from build123d import *

# Parameters (mm, degrees)
ESQUISSE1_R                  = 5
ESQUISSE1_R_2                = 4
ESQUISSE1_R_3                = 2
BOSS_EXTRU_1_DEPTH           = 5
ENL_V_MAT_EXTRU_1_DEPTH      = 1
ENL_V_MAT_EXTRU_1_DEPTH_BACK = 5
CONG_1_R                     = 10
ESQUISSE3_W                  = 20
ESQUISSE3_H                  = 5
BOSS_EXTRU_2_DEPTH           = 5
D_GAGEMENT_M21_D             = 2.4
D_GAGEMENT_M21_DEPTH         = 5
CONG_2_R                     = 10


with BuildPart() as part:
    # Esquisse1 → Boss.-Extru.1 (new body)
    with BuildSketch(Plane.XY):
        Polygon((0, 0), (30, 50), (50, 50), (50, 40), align=None)
        with Locations((36.602361653, 43.673429465)):
            Circle(ESQUISSE1_R, mode=Mode.SUBTRACT)
        with Locations((26.397486101, 32.05434035)):
            Circle(ESQUISSE1_R_2, mode=Mode.SUBTRACT)
        with Locations((18.668376917, 21.496804042)):
            Circle(ESQUISSE1_R_3, mode=Mode.SUBTRACT)
    extrude(amount=BOSS_EXTRU_1_DEPTH)

    # Esquisse2 → Enlèv. mat.-Extru.1 (cut, two sides)
    with BuildSketch(Plane(origin=(0, 0, 0), x_dir=(-1, 0, 0), z_dir=(0, 0, -1))) as enl_v_mat_extru_1_sk:
        with BuildLine():
            Line((0, 0), (-2.185666909, 3.642778182))
            ThreePointArc((-2.185666909, 3.642778182), (-2.607581993, 2.90339912), (-3.446178626, 2.756942901))
            Line((-3.446178626, 2.756942901), (0, 0))
        make_face()
    extrude(amount=ENL_V_MAT_EXTRU_1_DEPTH, mode=Mode.SUBTRACT)
    extrude(enl_v_mat_extru_1_sk.sketch, amount=-ENL_V_MAT_EXTRU_1_DEPTH_BACK, mode=Mode.SUBTRACT)

    # Congé1
    cong_1_edges = [part.edges().sort_by_distance(p)[0] for p in [
        (50, 40, 2.5),
    ]]
    fillet(cong_1_edges, radius=CONG_1_R)

    # Esquisse3 → Boss.-Extru.2 (add)
    with BuildSketch(Plane(origin=(0, 50, 0), x_dir=(1, 0, 0), z_dir=(0, 1, 0))):
        with Locations((40, -2.5)):
            Rectangle(ESQUISSE3_W, ESQUISSE3_H)
    extrude(amount=BOSS_EXTRU_2_DEPTH)

    # Dégagement M21
    with Locations(Plane.XY.offset(5)):
        with Locations((46, 52), (34, 52)):
            Hole(D_GAGEMENT_M21_D / 2, depth=D_GAGEMENT_M21_DEPTH)

    # Congé2
    cong_2_edges = [part.edges().sort_by_distance(p)[0] for p in [
        (30, 50, 2.5),
    ]]
    fillet(cong_2_edges, radius=CONG_2_R)


solid = part.part
Part model, mm, in its own coordinate system. A direction names the side the tool comes from. Round coordinates to 2 decimals unless told otherwise and drop trailing zeros. Write each loop counter-clockwise with the first axis right and the second up, starting at its lowest first coordinate (ties: lowest second). Pieces come first, ordered by that corner, then holes. Notation, with made-up numbers: M 7,78 L 24,78 A19 ccw 24,82 Z; hole C 88,-33.75 d4. An arc over 180 degrees is marked long. Return JSON: item names as keys, results as strings. Group by question number.
(1) Pin check, flat tips, straight feed: pin 1 Ø1.9 at (x, y) = (46, 52) entering from +Z; pin 2 Ø6.5 at (x, y) = (18.67, 21.5) entering from +Z; pin 3 Ø0.7 at (y, z) = (53.5, 1.5) entering from -X; pin 4 Ø2 at (x, z) = (7.5, 2.5) entering from -Y. Stop position of each tip, or through.
(2) Drill centre lines: probe 1 along Y at (x, z) = (33, 4.7); probe 2 along Y at (x, z) = (34, 1.8); probe 3 along Y at (x, z) = (32, 0.9). Where is each one in solid material? Low to high.
(3) Saw through at B-B on x = 28. Write the cut outline in (y, z).
(4) Saw through at A-A on y = 42. Write the cut outline in (x, z).
(5) Saw through at D-D on x = 33.5. Write the cut outline in (y, z), then the cut area to 3 significant figures.
(6) Saw through at C-C on z = 3.95. Write the cut outline in (x, y), then the cut area to 3 significant figures.
(7) Two-plate mould, pull along Y, no slides. Class faces 3 (the face through (31, 35, 5)), 4 (the face through (44.855, 52.36, 2.465)), 5 (the face through (25, 20, 2)): +Y half, -Y half, draft (parallel to the pull), parting line (faces both ways), or undercut.
(8) Which spindle directions (+Z, -Z, +X, -X, +Y, -Y) get a long thin tool onto all of the face, cutting with end or side? Do faces 1 (the face through (30, 54, 3)), 2 (the face through (31, 35, 0)). Say none if no direction does.
Returned:
{
 "1": {"pin 1": "through", "pin 2": "z = 5", "pin 3": "x = 30", "pin 4": "y = 5.2"},
 "2": {"probe 1": "26.4 to 40.21, 47.14 to 51.34, 52.66 to 55", "probe 2": "27.2 to 39.4, 47.94 to 50.8, 53.2 to 55", "probe 3": "25.6 to 41.72, 45.63 to 55"},
 "3": {"outline": "M 22.4,0 L 28.39,0 L 28.39,5 L 22.4,5 Z; M 35.72,0 L 46.67,0 L 46.67,5 L 35.72,5 Z"},
 "4": {"outline": "M 25.2,0 L 31.89,0 L 31.89,5 L 25.2,5 Z; M 41.31,0 L 49.6,0 L 49.6,5 L 41.31,5 Z"},
 "5": {"outline": "M 26.8,0 L 39.75,0 L 39.75,5 L 26.8,5 Z; M 47.59,0 L 50.91,0 L 50.91,5 L 47.59,5 Z; M 53.09,0 L 55,0 L 55,5 L 53.09,5 Z", "area": "90.9 mm²"},
 "6": {"outline": "M 2.19,3.64 A1 ccw 3.45,2.76 L 46.25,37 A10 ccw 50,44.81 L 50,55 L 30,55 L 30,52.77 A10 cw 28.57,47.62 Z; hole C 18.67,21.5 d4; hole C 26.4,32.05 d8; hole C 36.6,43.67 d10; hole C 34,52 d2.4; hole C 46,52 d2.4", "area": "694 mm²"},
 "7": {"face 3": "draft", "face 4": "undercut", "face 5": "-Y half"},
 "8": {"face 1": "+Z, -Z, -X, +Y", "face 2": "-Z, +X, -X, +Y, -Y"}
}
